```python
from build123d import *

# Parameters (mm, degrees)
SKETCH1_W               = 190
SKETCH1_H               = 120
SKETCH1_R               = 1.575
SKETCH1_R_2             = 1.7
SKETCH1_R_3             = 10.875
SKETCH1_R_4             = 10.75
SKETCH1_R_5             = 4.5
SKETCH1_R_6             = 6.2
BOSS_EXTRUDE1_DEPTH     = 5
SKETCH5_W               = 190
SKETCH5_H               = 120
CUT_EXTRUDE3_DEPTH      = 2
CUT_EXTRUDE3_DEPTH_BACK = 1
FILLET1_R               = 1
SKETCH6_R               = 1.875
CUT_EXTRUDE4_DEPTH      = 2.5


with BuildPart() as part:
    # Sketch1 → Boss-Extrude1 (new body)
    with BuildSketch(Plane.XY):
        Rectangle(SKETCH1_W, SKETCH1_H)
        with Locations((-91.5, 56.5)):
            Circle(SKETCH1_R, mode=Mode.SUBTRACT)
        with Locations((91.5, 56.5)):
            Circle(SKETCH1_R, mode=Mode.SUBTRACT)
        with Locations((91.5, -56.5)):
            Circle(SKETCH1_R, mode=Mode.SUBTRACT)
        with Locations((-91.5, -56.5)):
            Circle(SKETCH1_R, mode=Mode.SUBTRACT)
        with Locations((-36, 16)):
            Circle(SKETCH1_R_2, mode=Mode.SUBTRACT)
        with Locations((-36, -16)):
            Circle(SKETCH1_R_2, mode=Mode.SUBTRACT)
        with Locations((-68, -16)):
            Circle(SKETCH1_R_2, mode=Mode.SUBTRACT)
        with Locations((-68, 16)):
            Circle(SKETCH1_R_2, mode=Mode.SUBTRACT)
        with Locations((63, 28)):
            Circle(SKETCH1_R_3, mode=Mode.SUBTRACT)
        with Locations((0, -28)):
            Circle(SKETCH1_R_4, mode=Mode.SUBTRACT)
        with Locations((63, -28)):
            Circle(SKETCH1_R_5, mode=Mode.SUBTRACT)
        with Locations((-10, 38)):
            Circle(SKETCH1_R_6, mode=Mode.SUBTRACT)
        with Locations((10, 18)):
            Circle(SKETCH1_R_6, mode=Mode.SUBTRACT)
        with Locations((0, -2)):
            Circle(SKETCH1_R_6, mode=Mode.SUBTRACT)
        with Locations((-10, 18)):
            Circle(SKETCH1_R_6, mode=Mode.SUBTRACT)
        with Locations((10, 38)):
            Circle(SKETCH1_R_6, mode=Mode.SUBTRACT)
        with BuildLine():
            Line((-53, 8.645421567), (-53, 15.954278592))
            ThreePointArc((-53, 15.954278592), (-63.303517271, 11.303517271), (-67.954278592, 1))
            Line((-67.954278592, 1), (-60.645421567, 1))
            ThreePointArc((-60.645421567, 1), (-58.153995209, 6.153995209), (-53, 8.645421567))
        make_face(mode=Mode.SUBTRACT)
        with BuildLine():
            Line((-51, 8.645421567), (-51, 15.954278592))
            ThreePointArc((-51, 15.954278592), (-40.696482729, 11.303517271), (-36.045721408, 1))
            Line((-36.045721408, 1), (-43.354578433, 1))
            ThreePointArc((-43.354578433, 1), (-45.846004791, 6.153995209), (-51, 8.645421567))
        make_face(mode=Mode.SUBTRACT)
        with BuildLine():
            Line((-43.354578433, -1), (-36.045721408, -1))
            ThreePointArc((-36.045721408, -1), (-40.696482729, -11.303517271), (-51, -15.954278592))
            Line((-51, -15.954278592), (-51, -8.645421567))
            ThreePointArc((-51, -8.645421567), (-45.846004791, -6.153995209), (-43.354578433, -1))
        make_face(mode=Mode.SUBTRACT)
        with BuildLine():
            Line((-53, -8.645421567), (-53, -15.954278592))
            ThreePointArc((-53, -15.954278592), (-63.303517271, -11.303517271), (-67.954278592, -1))
            Line((-67.954278592, -1), (-60.645421567, -1))
            ThreePointArc((-60.645421567, -1), (-58.153995209, -6.153995209), (-53, -8.645421567))
        make_face(mode=Mode.SUBTRACT)
    extrude(amount=BOSS_EXTRUDE1_DEPTH)

    # Sketch5 → Cut-Extrude3 (cut, two sides)
    with BuildSketch(Plane.XY) as cut_extrude3_sk:
        Rectangle(SKETCH5_W, SKETCH5_H)
        Polygon((-87.5, 57.5), (87.5, 57.5), (87.5, 52.5), (92.5, 52.5), (92.5, -52.5), (87.5, -52.5), (87.5, -57.5), (-87.5, -57.5), (-87.5, -52.5), (-92.5, -52.5), (-92.5, 52.5), (-87.5, 52.5), align=None, mode=Mode.SUBTRACT)
    extrude(amount=CUT_EXTRUDE3_DEPTH, mode=Mode.SUBTRACT)
    extrude(cut_extrude3_sk.sketch, amount=-CUT_EXTRUDE3_DEPTH_BACK, mode=Mode.SUBTRACT)

    # Fillet1
    fillet1_edges = [part.edges().sort_by_distance(p)[0] for p in [
        (-43.354578433, -1, 2.5),
        (-51, -8.645421567, 2.5),
        (-51, -15.954278592, 2.5),
        (-36.045721408, -1, 2.5),
        (-53, -8.645421567, 2.5),
        (-60.645421567, -1, 2.5),
        (-67.954278592, -1, 2.5),
        (-53, -15.954278592, 2.5),
        (-60.645421567, 1, 2.5),
        (-53, 8.645421567, 2.5),
        (-53, 15.954278592, 2.5),
        (-67.954278592, 1, 2.5),
        (-51, 8.645421567, 2.5),
        (-43.354578433, 1, 2.5),
        (-36.045721408, 1, 2.5),
        (-51, 15.954278592, 2.5),
    ]]
    fillet(fillet1_edges, radius=FILLET1_R)

    # Sketch6 → Cut-Extrude4 (cut)
    with BuildSketch(Plane(origin=(0, 0, 0), x_dir=(-1, 0, 0), z_dir=(0, 0, -1))):
        with Locations((-72.6, -28)):
            Circle(SKETCH6_R)
    extrude(amount=-CUT_EXTRUDE4_DEPTH, mode=Mode.SUBTRACT)


solid = part.part
```
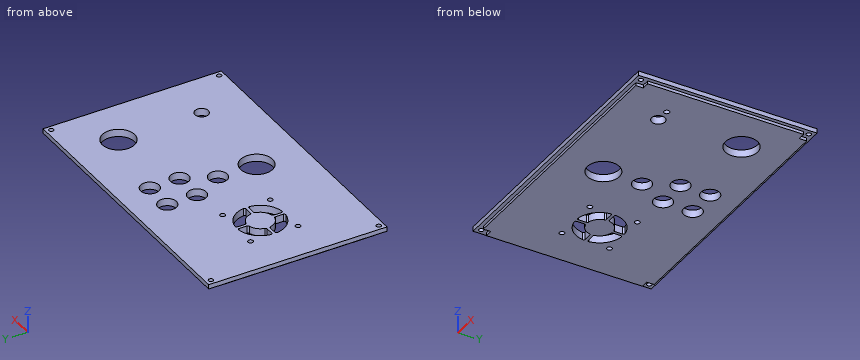
Geometry: final body of the model. Coordinates: model frame, mm. Round coordinates to 2 decimals unless told otherwise and drop trailing zeros. Order: outer loops, then holes, each group sorted by start corner. A loop starts at its lowest first (then second) coordinate and runs counter-clockwise, first axis right, second up. Notation, with made-up numbers: M 21,26.25 L 34,26.25 A26 cw 34,40.25 Z; hole C 52,-18 d1. An arc over 180 degrees is marked long. One line per item, written item: value.
(1) Line query: probe 1 along Y at (x, z) = (-36, 2.9); probe 2 along X at (y, z) = (-56.5, 3.85) (3 decimals); probe 3 along X at (y, z) = (-27.5, 4.75). Output: solid intervals per line, ascending. Write a range as [from, to].
Result sheet:
probe 1: [-60, -17.7], [-14.3, 14.3], [17.7, 60]
probe 2: [-95, -93.075], [-89.925, 89.925], [93.075, 95]
probe 3: [-95, -10.74], [10.74, 58.53], [67.47, 95]
(2) Cut plane A-A (x = 63). Return the cut outline in (y, z) (3 decimals).
Result sheet:
outline: M -60,2 L -57.5,2 L -57.5,0 L -32.5,0 L -32.5,5 L -60,5 Z; M -23.5,0 L 17.125,0 L 17.125,5 L -23.5,5 Z; M 38.875,0 L 57.5,0 L 57.5,2 L 60,2 L 60,5 L 38.875,5 Z
(3) Cut plane B-B (x = 44). Return the cut outline in (y, z).
Result sheet:
outline: M -60,2 L -57.5,2 L -57.5,0 L 57.5,0 L 57.5,2 L 60,2 L 60,5 L -60,5 Z
(4) Cut plane D-D (y = -19.5). Return the cut outline in (x, z), and give its area (3 significant figures).
Result sheet:
outline: M -95,2 L -92.5,2 L -92.5,0 L -6.58,0 L -6.58,5 L -95,5 Z; M 6.58,0 L 92.5,0 L 92.5,2 L 95,2 L 95,5 L 6.58,5 Z
area: 874 mm2
(5) Pin query (flat end, axial travel): P1, Ø12, axis at x = -13, y = -3.5, coming from the -Z side; P2, Ø1.5, axis at x = 20, z = 0.5, coming from the +Y side; P3, Ø19.5, axis at x = 63, y = 28, coming from the -Z side; P4, Ø1, axis at y = 56, z = 0.5, coming from the -X side. Return the tip coordinate at first contact, or that it passes through.
Result sheet:
P1: z = 0
P2: y = 57.5
P3: through
P4: x = -87.5
(6) Cut plane C-C (z = 3.35). Give the number of separate pieces and of enclosed holes in the cut face, and give its area (3 significant figures).
Result sheet:
separate pieces: 1
enclosed holes: 20
area: 20,800 mm2
